Design review of the part shown in the three views and the two pictorial views. Dimensions are in mm from the part's minimum x, y and z. Coordinates: 2 decimals unless noted, no trailing zeros. Write each loop counter-clockwise with the first axis right and the second up, starting at its lowest first coordinate (ties: lowest second). Pieces come first, ordered by that corner, then holes. Notation, with made-up numbers: M 76.25,81 L 133.25,81 A7 ccw 133.25,88 Z; hole C 45.5,13.25 d1. An arc over 180 degrees is marked long. Answer as a JSON object with one key per item and string values.
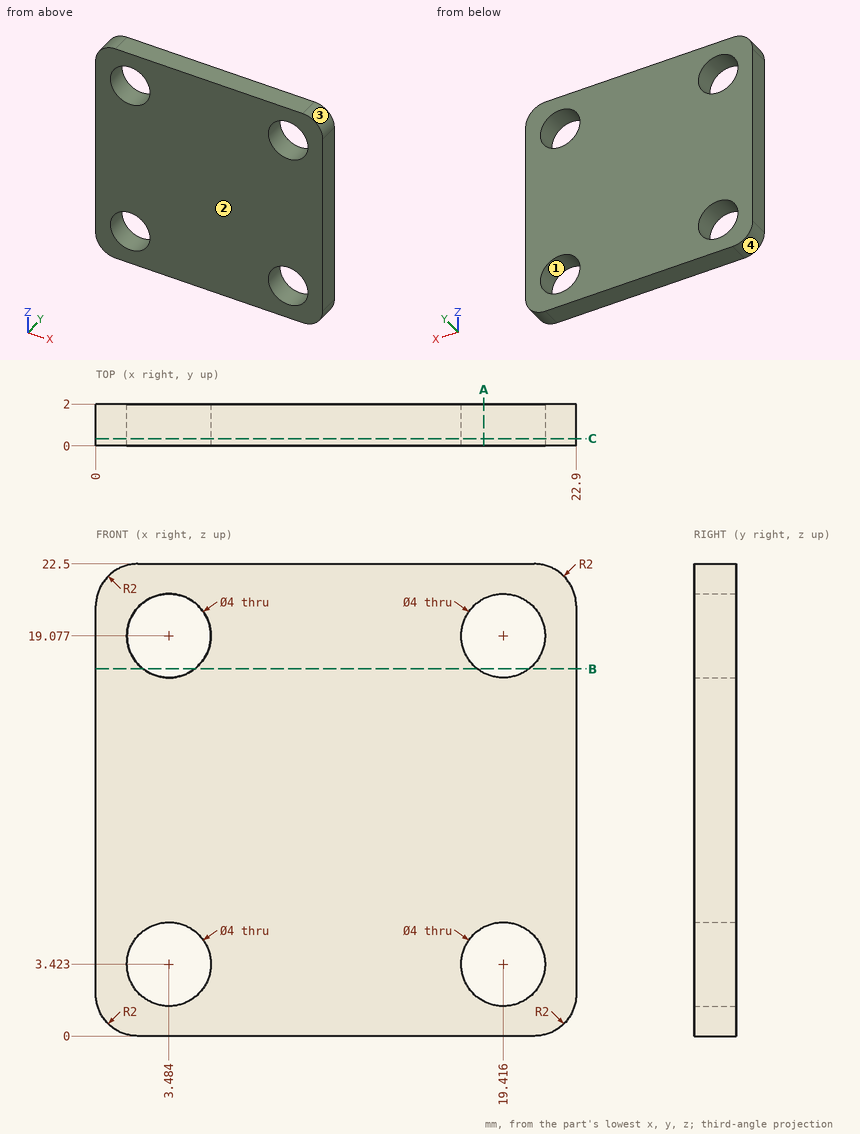
(1) For pin 1 Ø4 at (x, z) = (7, 16.5) entering from -Y; pin 2 Ø3 at (x, z) = (3.48, 3.42) entering from -Y, all flat-tipped, find the tip position at first contact; note any pin that passes through.
Results list:
{"pin 1": "y = 0", "pin 2": "through"}
(2) Draft analysis for pull direction X (two halves, no side actions). For the marked faces 1, 2, 3 and 4, state which applies: released by +X, released by -X, zero draft, split by the parting line, or undercut.
Results list:
{"face 1": "undercut", "face 2": "zero draft", "face 3": "released by +X", "face 4": "released by -X"}
(3) Wall thickness on line 1 along X through (y, z) = (0.3, 18.75); line 2 along X through (y, z) = (1.75, 19.75); line 3 along Z through (x, y) = (1.75, 1.65) (1 decimal): over which ranges is each line inside the solid? List them lowest first. Write a range as from..to.
Results list:
{"line 1": "0..1.51, 5.46..17.44, 21.39..22.9", "line 2": "0..1.6, 5.37..17.53, 21.3..22.9", "line 3": "0..2.4, 4.4..18.1, 20.1..22.5"}
(4) Add section C-C on y = 0.35. Give the boundary of the cut face in (x, z).
Results list:
{"outline": "M 0,2 A2 ccw 2,0 L 20.9,0 A2 ccw 22.9,2 L 22.9,20.5 A2 ccw 20.9,22.5 L 2,22.5 A2 ccw 0,20.5 Z; hole C 3.48,3.42 d4; hole C 3.48,19.08 d4; hole C 19.42,3.42 d4; hole C 19.42,19.08 d4"}
(5) Add section B-B on z = 17.5. Give the boundary of the cut face in (x, y).
Results list:
{"outline": "M 0,0 L 2.25,0 L 2.25,2 L 0,2 Z; M 4.71,0 L 18.19,0 L 18.19,2 L 4.71,2 Z; M 20.65,0 L 22.9,0 L 22.9,2 L 20.65,2 Z"}
(6) Add section A-A on x = 18.5. Give the boundary of the cut face in (y, z) (1 decimal).
Results list:
{"outline": "M 0,0 L 2,0 L 2,1.6 L 0,1.6 Z; M 0,5.2 L 2,5.2 L 2,17.3 L 0,17.3 Z; M 0,20.9 L 2,20.9 L 2,22.5 L 0,22.5 Z"}
